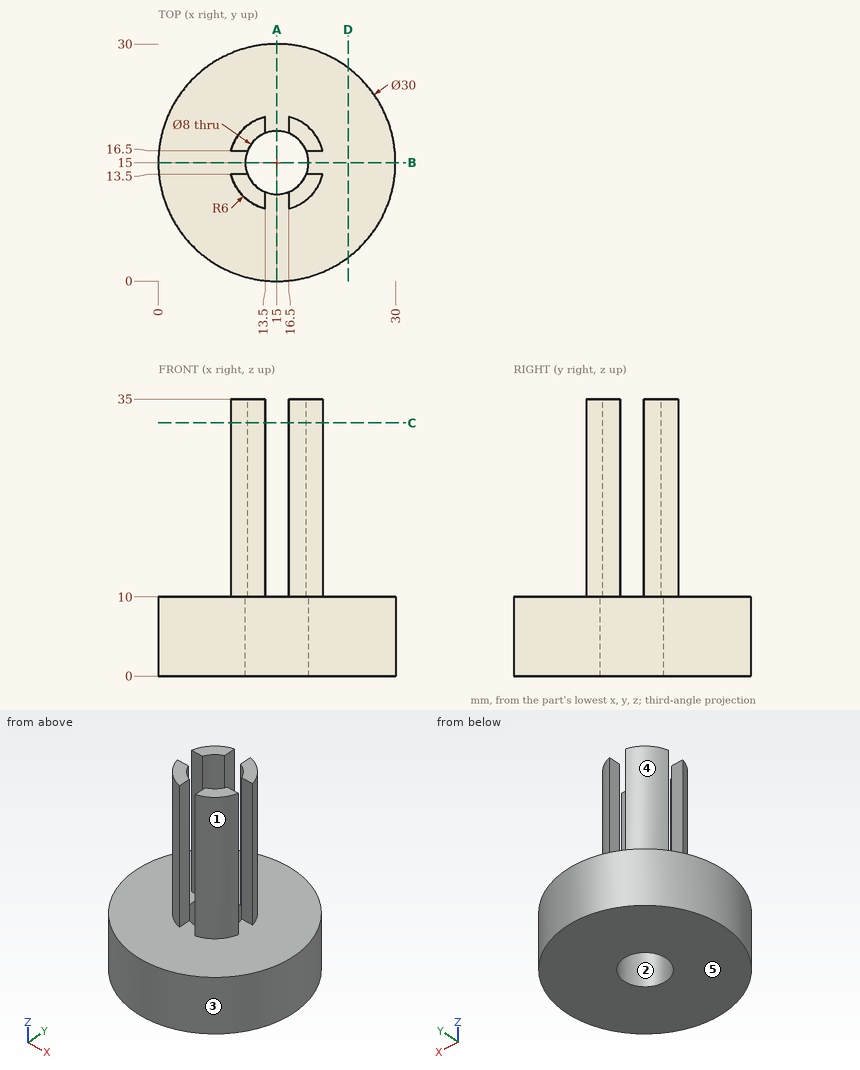
Geometry check sheet. Reference: drawing and pictorial views, mm from the part's lowest x, y, z. A direction names the side the tool comes from. Coordinates: 2 decimals unless noted, no trailing zeros. Order: outer loops, then holes, each group sorted by start corner. A loop starts at its lowest first (then second) coordinate and runs counter-clockwise, first axis right, second up. Notation, with made-up numbers: (-34.5, -30) -> (-15.5, -30) arc R6 ccw to (-15.5, -21) -> close; hole circle Ø1 at (-33.75, 53.25). An arc over 180 degrees is marked (long way). Put each result on its own line as item: value. Start each with the question number.
1) Tool access check on the marked faces 4 and 5. Record the directions out of +Z, -Z, +X, -X, +Y, -Y that give a thin tool (end or side, any length) a straight path to the whole face; none if there is none.
2) Cross-section at C-C (z = 32). Enter the section's corners in (x, y), plus the area to 3 significant figures.
3) Go/stop test with flat-tipped pins: pin 1 (1.7 mm diameter, centred on y = 10.5, z = 26.5, fed in from -X); pin 2 (1.7 mm diameter, centred on y = 20.5, z = 19.5, fed in from -X); pin 3 (2.5 mm diameter, centred on x = 10, z = 16.5, fed in from +Y); pin 4 (8 mm diameter, centred on x = 8.5, y = 23, fed in from -Z). Record where each tip stops, or that it passes through.
4) Cross-section at D-D (x = 24). Enter the section's corners in (y, z).
5) Release check for a two-part mould opening along Y. For the marked faces 1, 2 and 3 record: pulls with the +Y half, pulls with the -Y half, needs draft (parallel to the pull), parting line crosses it, or undercut.
6) Material ranges on L1, parallel to X at y = 12, z = 20; L2, parallel to Z at x = 25.25, y = 12; L3, parallel to Y at x = 18.5, z = 3, recorded low to high.
7) Cross-section at A-A (x = 15). Enter the section's corners in (y, z).
Geometry check:
1. face 4: +Z, -X, +Y
1. face 5: -Z, +X, -X, +Y, -Y
2. outline: (9.19, 13.5) arc R6 ccw to (13.5, 9.19) -> (13.5, 11.29) arc R4 cw to (11.29, 13.5) -> close; (9.19, 16.5) -> (11.29, 16.5) arc R4 cw to (13.5, 18.71) -> (13.5, 20.81) arc R6 ccw to start; (16.5, 9.19) arc R6 ccw to (20.81, 13.5) -> (18.71, 13.5) arc R4 cw to (16.5, 11.29) -> close; (16.5, 18.71) arc R4 cw to (18.71, 16.5) -> (20.81, 16.5) arc R6 ccw to (16.5, 20.81) -> close
2. area: 38.4 mm^2
3. pin 1: stops at x = 10.24
3. pin 2: stops at x = 11.21
3. pin 3: stops at y = 19.68
3. pin 4: stops at z = 0
4. outline: (3, 0) -> (27, 0) -> (27, 10) -> (3, 10) -> close
5. face 1: pulls with the -Y half
5. face 2: undercut
5. face 3: parting line crosses it
6. L1: x = 9.8 to 12.35, 17.65 to 20.2
6. L2: z = 0 to 10
6. L3: y = 0.41 to 13.06, 16.94 to 29.59
7. outline: (0, 0) -> (11, 0) -> (11, 10) -> (0, 10) -> close; (19, 0) -> (30, 0) -> (30, 10) -> (19, 10) -> close
